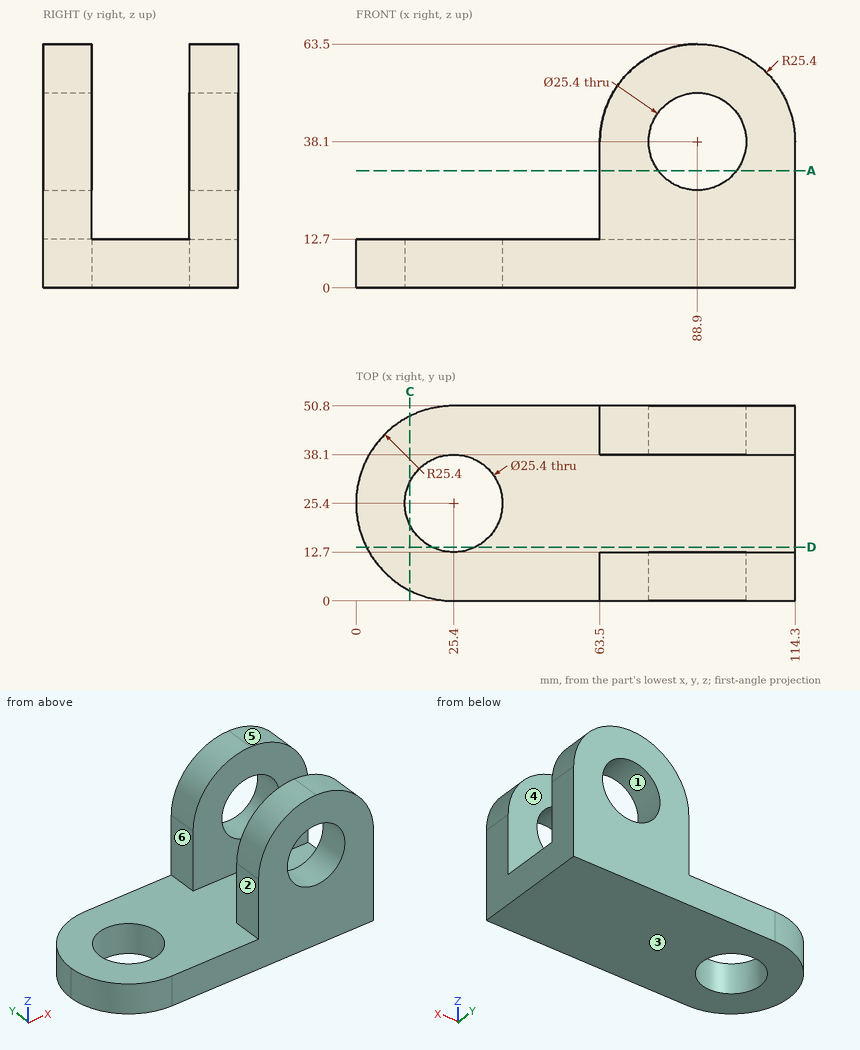
Source: three-view drawing plus pictorial views. Frame: mm from the lowest corner of the part. A direction names the side the tool comes from. Round coordinates to 2 decimals unless told otherwise and drop trailing zeros. Order: outer loops, then holes, each group sorted by start corner. A loop starts at its lowest first (then second) coordinate and runs counter-clockwise, first axis right, second up. Notation, with made-up numbers: M 54,79 L 70,79 A35 cw 70,113 Z; hole C 58,1.5 d5. An arc over 180 degrees is marked long. One line per item, written item: value.
(1) Pull-direction query (X, two-part tool) for the marked faces 1, 2 and 3; classes: pulls with the +X half, pulls with the -X half, needs draft (parallel to the pull), parting line crosses it, or undercut.
Result sheet:
face 1: undercut
face 2: pulls with the -X half
face 3: needs draft
(2) Line query: probe 1 along Y at (x, z) = (100.5, 32); probe 2 along Z at (x, y) = (89, 45); probe 3 along X at (y, z) = (25, 3). Output: solid intervals per line, ascending. Write a range as [from, to].
Result sheet:
probe 1: [0, 12.7], [38.1, 50.8]
probe 2: [0, 25.4], [50.8, 63.5]
probe 3: [0, 12.71], [38.09, 114.3]
(3) Cut plane D-D (y = 14). Return the cut outline in (x, z), and give its area (3 significant figures).
Result sheet:
outline: M 2.7,0 L 19.8,0 L 19.8,12.7 L 2.7,12.7 Z; M 31,0 L 114.3,0 L 114.3,12.7 L 31,12.7 Z
area: 1,280 mm2
(4) Cut plane A-A (z = 30.5). Return the cut outline in (x, y), and give its area (3 significant figures).
Result sheet:
outline: M 63.5,0 L 78.73,0 L 78.73,12.7 L 63.5,12.7 Z; M 63.5,38.1 L 78.73,38.1 L 78.73,50.8 L 63.5,50.8 Z; M 99.07,0 L 114.3,0 L 114.3,12.7 L 99.07,12.7 Z; M 99.07,38.1 L 114.3,38.1 L 114.3,50.8 L 99.07,50.8 Z
area: 773 mm2
(5) Pin query (flat end, axial travel): P1, Ø4, axis at y = 44.5, z = 29.5, coming from the -X side; P2, Ø4, axis at x = 64.5, y = 13, coming from the +Z side; P3, Ø10, axis at y = 8, z = 53, coming from the -X side. Return the tip coordinate at first contact, or that it passes through.
Result sheet:
P1: x = 63.5
P2: z = 50.03
P3: x = 65.51
(6) Reachability of the marked faces 4, 5 and 6 from +Z, -Z, +X, -X, +Y, -Y: full face, straight path, thin tool, end or side. Return the list, or none.
Result sheet:
face 4: +Z, +X, -X
face 5: +Z, +X, +Y, -Y
face 6: +Z, -X, +Y, -Y
(7) Cut plane C-C (x = 14). Return the cut outline in (y, z).
Result sheet:
outline: M 2.7,0 L 19.8,0 L 19.8,12.7 L 2.7,12.7 Z; M 31,0 L 48.1,0 L 48.1,12.7 L 31,12.7 Z
